Read the model definition and answer for the solid it produces. Units are mm, in the model's axes. Coordinates: 2 decimals unless noted, no trailing zeros. Order: outer loops, then holes, each group sorted by start corner. A loop starts at its lowest first (then second) coordinate and runs counter-clockwise, first axis right, second up. Notation, with made-up numbers: M -13.5,-2 L 12.5,-2 A20 cw 12.5,8 Z; hole C 58,40 d4. An arc over 180 degrees is marked long. Write each question's results on one line, items separated by ' | '.
```python
from build123d import *

# Parameters (mm, degrees)
F0_W     = 152.4
F0_H     = 15.24
F1_DEPTH = 2.54
F2_R     = 5.08
F3_R     = 3.180059
F4_DEPTH = 25.4


with BuildPart() as f1:
    # F0 (on Front) → F1 (new body)
    with BuildSketch(Plane.XZ):
        Rectangle(F0_W, F0_H)
    extrude(amount=F1_DEPTH)

    # F2
    f2_edges = [f1.edges().sort_by_distance(p)[0] for p in [
        (-76.2, -1.27, 7.62),
        (-76.2, -1.27, -7.62),
        (76.2, -1.27, 7.62),
        (76.2, -1.27, -7.62),
    ]]
    fillet(f2_edges, radius=F2_R)

    # F3 (on face) → F4 (cut)
    with BuildSketch(Plane.XZ.offset(2.54)):
        with Locations((-70.363984, 0)):
            Circle(F3_R)
        with Locations((70.363984, 0)):
            Circle(F3_R)
    extrude(amount=-F4_DEPTH, mode=Mode.SUBTRACT)


solid = f1.part
```
(1) The part is cut by section C-C, the plane z = -6. Write down the section's boundary in (x, y).
Conclusion:
outline: M -74.84,-2.54 L 74.84,-2.54 L 74.84,0 L -74.84,0 Z
(2) The part is cut by section B-B, the plane z = 0. Write down the section's boundary in (x, y), then the cut area to 3 significant figures.
Conclusion:
outline: M -76.2,-2.54 L -73.54,-2.54 L -73.54,0 L -76.2,0 Z; M -67.18,-2.54 L 67.18,-2.54 L 67.18,0 L -67.18,0 Z; M 73.54,-2.54 L 76.2,-2.54 L 76.2,0 L 73.54,0 Z | area: 355 mm²
(3) Straight lines are drawn through the part: line 1 (X direction, y = -0.8, z = 2.5); line 2 (X direction, y = -1.2, z = 2); line 3 (X direction, y = -1.9, z = 7). For each, find the intervals that lie inside material, in ascending order.
Conclusion:
line 1: -76.2 to -72.33, -68.4 to 68.4, 72.33 to 76.2 | line 2: -76.2 to -72.84, -67.89 to 67.89, 72.84 to 76.2 | line 3: -73.55 to 73.55
(4) The mould has two halves that part along Z. Classify faces 1 (the flat face through (-1, 0, 0)), 2 (the cylindrical face through (73.3, -1.29, -1.22)), 3 (the cylindrical face through (-74.751, -1.288, 6.092)): pulls with the +Z half, pulls with the -Z half, needs draft (parallel to the pull), parting line crosses it, or undercut.
Conclusion:
face 1: needs draft | face 2: undercut | face 3: pulls with the +Z half
(5) The part is cut by section A-A, the plane y = -2.1. Write down the section's boundary in (x, z), then the cut area to 3 significant figures.
Conclusion:
outline: M -76.2,-2.54 A5.08 ccw -71.12,-7.62 L 71.12,-7.62 A5.08 ccw 76.2,-2.54 L 76.2,2.54 A5.08 ccw 71.12,7.62 L -71.12,7.62 A5.08 ccw -76.2,2.54 Z; hole C -70.36,0 d6.36; hole C 70.36,0 d6.36 | area: 2,240 mm²
(6) Given pin 1 (4 mm diameter, centred on x = 35.5, z = -2.5, fed in from +Y); pin 2 (1.5 mm diameter, centred on y = -1.5, z = -3.5, fed in from +X), each flat-ended and moving along its own axis, determine where each tip first touches the part or whether it passes through.
Conclusion:
pin 1: y = 0 | pin 2: x = 76.2
